Part model, mm, in its own coordinate system. Round coordinates to 2 decimals unless told otherwise and drop trailing zeros. Order: outer loops, then holes, each group sorted by start corner. A loop starts at its lowest first (then second) coordinate and runs counter-clockwise, first axis right, second up. Notation, with made-up numbers: M 20.5,17 L 38.5,17 A14 cw 38.5,26 Z; hole C 72,24 d3. An arc over 180 degrees is marked long. Write each question's results on one line, items separated by ' | '. Start each with the question number.
1. Band-saw the part on B-B, the plane z = -52. List the corners of the cut face in (x, y), then the cut area to 3 significant figures.
2. Band-saw the part on C-C, the plane x = 73. List the corners of the cut face in (y, z), then the cut area to 3 significant figures.
3. Drop flat-ended pins along their axis: pin 1 Ø0.5 at (x, y) = (150, 1) entering from -Z; pin 2 Ø5 at (x, z) = (449.28, -6.35) entering from +Y; pin 3 Ø0.8 at (x, y) = (126.5, 0.5) entering from +Z. Give the stop position or say it passes through.
4. Probe L1, parallel to Z at x = 12.7, y = 1.05; L2, parallel to X at y = 0.4, z = -55; L3, parallel to Z at x = 130.5, y = 0.1. List the from-to ranges inside material, lowest first. Write a range as [from, to].
5. Band-saw the part on A-A, the plane y = 0.5. Give the number of separate pieces and of enclosed holes in the cut face, then the cut area to 3 significant figures.
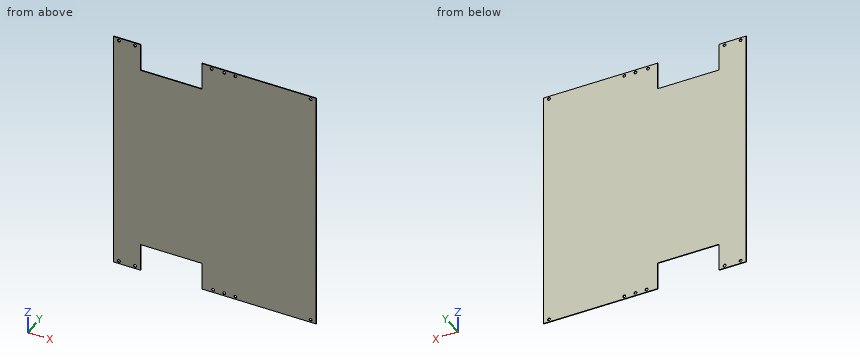
Autodesk Inventor part; units mm, degrees
ref_plane "YZ Plane" through (0, 0, 0) normal (1, 0, 0) x (0, 1, 0)
ref_plane "XZ Plane" through (0, 0, 0) normal (0, 1, 0) x (-1, 0, 0)
ref_plane "XY Plane" through (0, 0, 0) normal (0, 0, 1) x (1, 0, 0)
sketch "Sketch1" plane through (0, 0, 0) normal (0, 1, 0) x (-1, 0, 0)
  point P0 (0, 0)
sketch "Sketch2" plane through (0, 0, 0) normal (0, 1, 0) x (-1, 0, 0)
  line L0 (-61.9252, 0) -> (0, 0)
  line L1 (0, 0) -> (0, -558.8)
  line L2 (0, -558.8) -> (-61.9252, -558.8)
  line L3 (-61.9252, -558.8) -> (-61.9252, -495.3)
  line L4 (-61.9252, -495.3) -> (-201.6252, -495.3)
  line L5 (-201.6252, -495.3) -> (-201.6252, -558.8)
  line L6 (-201.6252, -558.8) -> (-461.9752, -558.8)
  line L7 (-461.9752, -558.8) -> (-461.9752, 0)
  line L8 (-461.9752, 0) -> (-201.6252, 0)
  line L9 (-201.6252, 0) -> (-201.6252, -63.5)
  line L10 (-201.6252, -63.5) -> (-61.9252, -63.5)
  line L11 (-61.9252, -63.5) -> (-61.9252, 0)
  point P0 (0, 0)
  dimension "d1" = 558.8
  dimension "d2" = 139.7
  dimension "d3" = 61.9252
  dimension "d4" = 63.5
  dimension "d8" = 260.35
extrude "Extrusion1" add sketch "Sketch2" along normal blind 1.5875
sketch "Sketch3" plane through (0, 1.5875, 0) normal (0, 1, 0) x (1, 0, 0)
  line L0 (461.9752, 0) -> (461.9752, 558.8)
  line L1 (461.9752, 0) -> (461.9752, 12.7)
  line L2 (461.9752, 12.7) -> (201.6252, 12.7)
  line L3 (201.6252, 63.5) -> (201.6252, 0)
  line L4 (201.6252, 558.8) -> (461.9752, 558.8)
  line L5 (461.9752, 558.8) -> (461.9752, 546.1)
  line L6 (461.9752, 546.1) -> (201.6252, 546.1)
  line L7 (201.6252, 558.8) -> (201.6252, 495.3)
  line L8 (461.9752, 6.35) -> (201.6252, 6.35)
  line L9 (461.9752, 552.45) -> (201.6252, 552.45)
  line L10 (461.9752, 552.45) -> (449.2752, 552.45)
  line L11 (461.9752, 6.35) -> (449.2752, 6.35)
  line L12 (201.6252, 552.45) -> (227.0252, 552.45)
  line L13 (227.0252, 552.45) -> (252.4252, 552.45)
  line L14 (252.4252, 552.45) -> (277.8252, 552.45)
  line L15 (201.6252, 6.35) -> (227.0252, 6.35)
  line L16 (227.0252, 6.35) -> (252.4252, 6.35)
  line L17 (252.4252, 6.35) -> (277.8252, 6.35)
  line L18 (0, 558.8) -> (0, 0)
  line L19 (0, 552.45) -> (62.0515, 552.45)
  line L20 (0, 6.35) -> (62.0515, 6.35)
  line L21 (0, 552.45) -> (12.7, 552.45)
  line L22 (61.9252, 495.3) -> (61.9252, 558.8)
  line L23 (61.9252, 552.45) -> (49.2252, 552.45)
  circle A0 centre (49.2252, 552.45) radius 3.2512
  circle A1 centre (12.7, 552.45) radius 3.2512
  circle A2 centre (227.0252, 552.45) radius 3.2512
  circle A3 centre (252.4252, 552.45) radius 3.2512
  circle A4 centre (277.8252, 552.45) radius 3.2512
  circle A5 centre (449.2752, 552.45) radius 3.2512
  line L24 (461.9752, 6.35) -> (449.2752, 6.35)
  circle A6 centre (449.2752, 6.35) radius 3.2512
  line L25 (201.6252, 6.35) -> (227.0252, 6.35)
  circle A7 centre (223.774, 6.35) radius 3.2512
  circle A8 centre (252.4252, 6.35) radius 3.2512
  circle A9 centre (277.8252, 6.35) radius 3.2512
  circle A10 centre (49.2252, 6.35) radius 3.2512
  circle A11 centre (12.7, 6.35) radius 3.2512
  line L26 (449.2752, 558.8) -> (449.2752, 0)
  line L27 (449.2752, 558.8) -> (455.6252, 558.8)
  line L28 (455.6252, 558.8) -> (455.6252, 0)
  line L29 (461.9752, 0) -> (201.6252, 0)
  line L30 (455.6252, 546.1) -> (455.6252, 368.3)
  line L31 (455.6252, 368.3) -> (455.6252, 190.5)
  circle A12 centre (455.6252, 368.3) radius 3.2512
  circle A13 centre (455.6252, 190.5) radius 3.2512
  dimension "d9" = 12.7
  dimension "d10" = 12.7
  dimension "d11" = 12.7
  dimension "d12" = 25.4
  dimension "d13" = 25.4
  dimension "d14" = 25.4
  dimension "d15" = 12.7
  dimension "d16" = 12.7
  dimension "d17" = 6.5024
  dimension "d18" = 12.7
  dimension "d19" = 177.8
  dimension "d20" = 177.8
  dimension "d21" = 6.5024
extrude "Extrusion2" cut sketch "Sketch3" against normal blind 25.4 contours A6 L26 L8 | L8 L26 A6 | A6 L8 L26 | L8 A6 L26 | A9 L8 | L8 A9 | A7 L8 | L8 A7 | A5 L26 L9 | L9 L26 A5 | A5 L9 L26 | L9 A5 L26 | A8 L8 | L8 A8 | A2 L9 | L9 A2 | A4 L9 | L9 A4 | A3 L9 | L9 A3 | A10 L20 | L20 A10 | A11 L20 | L20 A11 | A0 L19 | L19 A0 | A1 L19 | L19 A1
properties part number "Belly Pan" material "Aluminum 6061"
Solution:
1) outline: M 0,0 L 61.93,0 L 61.93,1.59 L 0,1.59 Z; M 201.63,0 L 461.98,0 L 461.98,1.59 L 201.63,1.59 Z | area: 512 mm^2
2) outline: M 0,-495.3 L 1.59,-495.3 L 1.59,-63.5 L 0,-63.5 Z | area: 685 mm^2
3) pin 1: z = -495.3 | pin 2: through | pin 3: z = -63.5
4) L1: [-558.8, -555.7], [-549.2, -9.6], [-3.1, 0] | L2: [0, 61.93], [201.63, 461.98] | L3: [-495.3, -63.5]
5) separate pieces: 1 | enclosed holes: 12 | area: 240,000 mm^2
